Autodesk Fusion 360 part; units mm, degrees
sketch "草图1" plane through (0, 0, 0) normal (0, 0, 1) x (1, 0, 0)
  circle A0 centre (0, 0) radius 4.25
  dimension "d1" = 8.5
extrude "拉伸1" add sketch "草图1" along normal blind 3.2
fillet "圆角1" radius 2 1 edges at (-3.9624, -1.5369, 3.2)
sketch "草图2" plane through (0, 0, 0) normal (0, 0, -1) x (1, 0, 0)
  circle A0 centre (0, 0) radius 4.25
  circle A1 centre (0, 0) radius 2.5
  dimension "d6" = 5
extrude "拉伸2" add sketch "草图2" along normal blind 25 contours A1
Build history of the part. All positions in model axes, mm. A direction names the side the tool comes from. Coordinates: 2 decimals unless noted, no trailing zeros. Order: outer loops, then holes, each group sorted by start corner. A loop starts at its lowest first (then second) coordinate and runs counter-clockwise, first axis right, second up. Notation, with made-up numbers: M -3,65 L 38,65 A15 cw 38,75 Z; hole C 40,82.5 d11. An arc over 180 degrees is marked long. One line per question, with ' | ' between items. Start each with the question number.
1. Cut at C-C (z = -0.5). Write the cut outline in (x, y), plus the area to 3 significant figures.
2. Cut at A-A (y = 0). Write the cut outline in (x, z).
3. Flat gauge pins, fed straight in: P1, Ø1, axis at y = -1, z = -9.5, coming from the -X side; P2, Ø1.5, axis at x = -2, z = -12.5, coming from the -Y side; P3, Ø5, axis at y = 1, z = -12.5, coming from the -X side. Where does each tip first touch, or does it go through?
4. Tool access for faces 1 (the face through (0, 0, 3.2)), 2 (the face through (-0.54, -2.44, -12.32)): list every direction of +Z, -Z, +X, -X, +Y, -Y with a clear straight run to the whole face (end or side of a thin tool).
5. Wall check: line 1 along Y through (x, z) = (0, -5); line 2 along Z through (x, y) = (1.5, 2.5). Give the ranges that are in metal, low to high. Write a range as [from, to].
The answers:
1) outline: C 0,0 d5 | area: 19.6 mm2
2) outline: M -4.25,0 L -2.5,0 L -2.5,-25 L 2.5,-25 L 2.5,0 L 4.25,0 L 4.25,1.2 A2 ccw 2.25,3.2 L -2.25,3.2 A2 ccw -4.25,1.2 Z
3) P1: stops at x = -2.45 | P2: stops at y = -2.17 | P3: stops at x = -2.5
4) face 1: +Z, +X, -X, +Y, -Y | face 2: -Z
5) line 1: y = [-2.5, 2.5] | line 2: z = [0, 3.09]
